Job drawing, mm, ordinate dimensions from the low corner. One solid piece. A direction names the side the tool comes from. Round coordinates to 2 decimals unless told otherwise and drop trailing zeros. Loops run counter-clockwise (first coordinate to the right, second up) from the corner with the lowest first, then second, coordinate; pieces in that order, holes last.
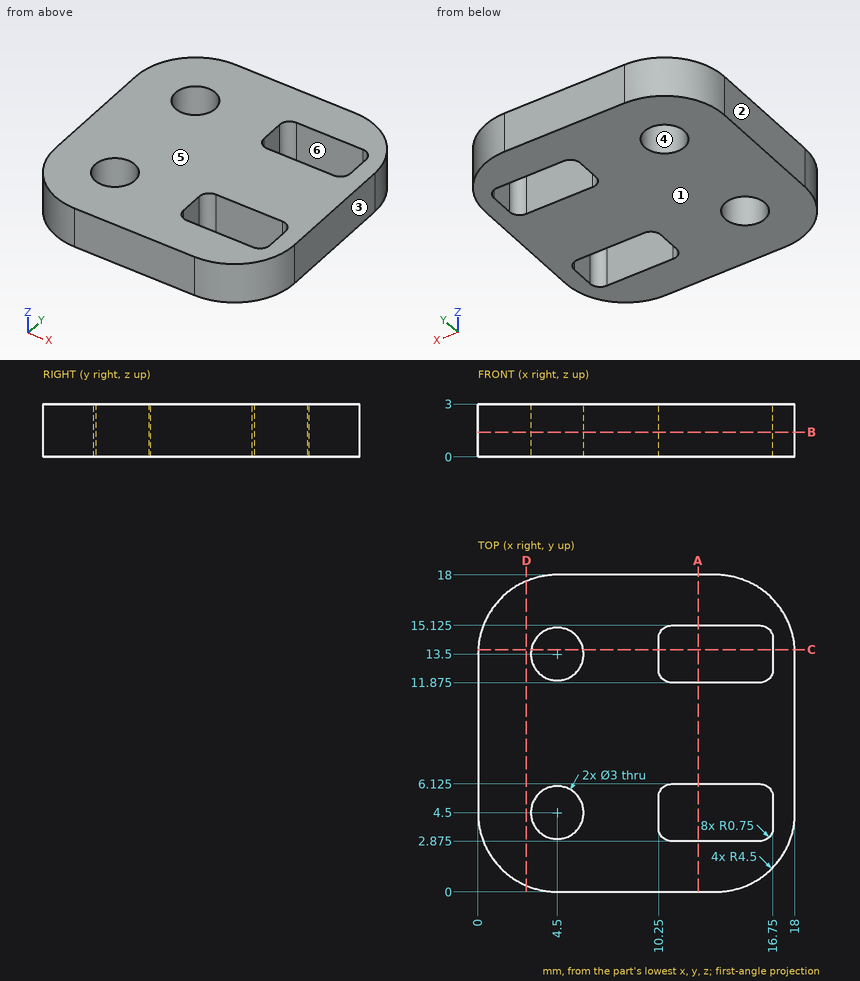
Item 1: Cut at C-C, the plane y = 13.75. Give the cut face in (x, z).
Answers follow:
outline: (0.01, 0) - (3.02, 0) - (3.02, 3) - (0.01, 3) - close; (5.98, 0) - (10.25, 0) - (10.25, 3) - (5.98, 3) - close; (16.75, 0) - (17.99, 0) - (17.99, 3) - (16.75, 3) - close
Item 2: Cut at D-D, the plane x = 2.75. Give the cut face in (y, z), plus the area to 3 significant figures.
Answers follow:
outline: (0.35, 0) - (17.65, 0) - (17.65, 3) - (0.35, 3) - close
area: 51.9 mm2
Item 3: Flat gauge pins, fed straight in: P1, Ø1.5, axis at x = 14, z = 1.5, coming from the +Y side; P2, Ø1.5, axis at x = 14.5, z = 2, coming from the -Y side; P3, Ø1, axis at y = 3.5, z = 1.5, coming from the -X side; P4, Ø2.5, axis at x = 4.5, y = 13.5, coming from the +Z side. Where does each tip first touch, or does it go through?
Answers follow:
P1: stops at y = 18
P2: stops at y = 0.01
P3: stops at x = 0.03
P4: passes through
Item 4: Probe line 1 (X direction, y = 13.5, z = 1.55); line 2 (Y direction, x = 11.5, z = 0.7) (3 decimals); line 3 (Y direction, x = 5.5, z = 2.15). List the from-to ranges inside material, lowest first.
Answers follow:
line 1: x = 0 to 3, 6 to 10.25, 16.75 to 18
line 2: y = 0 to 2.875, 6.125 to 11.875, 15.125 to 18
line 3: y = 0 to 3.38, 5.62 to 12.38, 14.62 to 18
Item 5: Two-plate mould, pull along X, no slides. Class the marked faces 1, 2, 3 and 4: released by +X, released by -X, zero draft, split by the parting line, or undercut.
Answers follow:
face 1: zero draft
face 2: released by -X
face 3: released by +X
face 4: undercut
Item 6: Cut at A-A, the plane x = 12.5. Give the cut face in (y, z) (3 decimals), plus the area to 3 significant figures.
Answers follow:
outline: (0, 0) - (2.875, 0) - (2.875, 3) - (0, 3) - close; (6.125, 0) - (11.875, 0) - (11.875, 3) - (6.125, 3) - close; (15.125, 0) - (18, 0) - (18, 3) - (15.125, 3) - close
area: 34.5 mm2
Item 7: Cut at B-B, the plane z = 1.4. Give the cut face in (x, y) (3 decimals), plus the area to 3 significant figures.
Answers follow:
outline: (0, 4.5) arc R4.5 ccw to (4.5, 0) - (13.5, 0) arc R4.5 ccw to (18, 4.5) - (18, 13.5) arc R4.5 ccw to (13.5, 18) - (4.5, 18) arc R4.5 ccw to (0, 13.5) - close; hole circle Ø3 at (4.5, 4.5); hole circle Ø3 at (4.5, 13.5); hole (10.25, 3.625) arc R0.75 ccw to (11, 2.875) - (16, 2.875) arc R0.75 ccw to (16.75, 3.625) - (16.75, 5.375) arc R0.75 ccw to (16, 6.125) - (11, 6.125) arc R0.75 ccw to (10.25, 5.375) - close; hole (10.25, 12.625) arc R0.75 ccw to (11, 11.875) - (16, 11.875) arc R0.75 ccw to (16.75, 12.625) - (16.75, 14.375) arc R0.75 ccw to (16, 15.125) - (11, 15.125) arc R0.75 ccw to (10.25, 14.375) - close
area: 251 mm2
Item 8: 3-axis set-ups, long thin cutter, end or side, ignore diameter. For the marked faces 5 and 6: which of +Z, -Z, +X, -X, +Y, -Y reach the whole face in a straight line?
Answers follow:
face 5: +Z, +X, -X, +Y, -Y
face 6: +Z, -Z
